```python
from build123d import *

# Parameters (mm, degrees)
F0_W     = 195.58
F0_H     = 127
F1_DEPTH = 2.54
F2_W     = 29.21
F2_H     = 2.54
F2_W_2   = 12.7
F2_H_2   = 12.7
F3_DEPTH = 2.54


with BuildPart() as f1:
    # F0 (on Front) → F1 (new body)
    with BuildSketch(Plane.XZ):
        Rectangle(F0_W, F0_H)
    extrude(amount=F1_DEPTH)

    # F2 (on face) → F3 (cut)
    with BuildSketch(Plane.XZ.offset(2.54)):
        with Locations((-31.369, -51.8922)):
            Rectangle(F2_W, F2_H)
        with Locations((19.304, -46.8122)):
            Rectangle(F2_W_2, F2_H_2)
        with Locations((55.118, -46.8122)):
            Rectangle(F2_W_2, F2_H_2)
    extrude(amount=-F3_DEPTH, mode=Mode.SUBTRACT)


solid = f1.part
```
Verification items for the finished model (mm, model axes). Give positions to 0.01 mm unless a question says otherwise; leave off trailing zeros. Order: outer loops, then holes, each group sorted by start corner. A loop starts at its lowest first (then second) coordinate and runs counter-clockwise, first axis right, second up. Notation, with made-up numbers: (-6, 85) -> (37, 85) arc R25 ccw to (37, 111) -> close; hole circle Ø7 at (35, 55). An arc over 180 degrees is marked (long way). Use a Markdown table: item, result.
1) Section check B-B, the plane y = -1.25. Record the boundary of the cut face in (x, z), then the cut area to 3 significant figures.
Results:
| item | result |
|---|---|
| outline | (-97.79, -63.5) -> (97.79, -63.5) -> (97.79, 63.5) -> (-97.79, 63.5) -> close; hole (-45.97, -53.16) -> (-16.76, -53.16) -> (-16.76, -50.62) -> (-45.97, -50.62) -> close; hole (12.95, -53.16) -> (25.65, -53.16) -> (25.65, -40.46) -> (12.95, -40.46) -> close; hole (48.77, -53.16) -> (61.47, -53.16) -> (61.47, -40.46) -> (48.77, -40.46) -> close |
| area | 24,400 mm² |
2) Section check A-A, the plane x = 21. Record the boundary of the cut face in (y, z).
Results:
| item | result |
|---|---|
| outline | (-2.54, -63.5) -> (0, -63.5) -> (0, -53.16) -> (-2.54, -53.16) -> close; (-2.54, -40.46) -> (0, -40.46) -> (0, 63.5) -> (-2.54, 63.5) -> close |
3) Section check C-C, the plane x = -27.5. Record the boundary of the cut face in (y, z).
Results:
| item | result |
|---|---|
| outline | (-2.54, -63.5) -> (0, -63.5) -> (0, -53.16) -> (-2.54, -53.16) -> close; (-2.54, -50.62) -> (0, -50.62) -> (0, 63.5) -> (-2.54, 63.5) -> close |
4) Material ranges on probe 1 along X at (y, z) = (-1.4, -46.5); probe 2 along X at (y, z) = (-2, -52.5); probe 3 along Z at (x, y) = (-27, -2.15), recorded low to high.
Results:
| item | result |
|---|---|
| probe 1 | -97.79 to 12.95, 25.65 to 48.77, 61.47 to 97.79 |
| probe 2 | -97.79 to -45.97, -16.76 to 12.95, 25.65 to 48.77, 61.47 to 97.79 |
| probe 3 | -63.5 to -53.16, -50.62 to 63.5 |
